Autodesk Inventor part; units mm, degrees
ref_plane "YZ Plane" through (0, 0, 0) normal (1, 0, 0) x (0, 1, 0)
ref_plane "XZ Plane" through (0, 0, 0) normal (0, 1, 0) x (-1, 0, 0)
ref_plane "XY Plane" through (0, 0, 0) normal (0, 0, 1) x (1, 0, 0)
sketch "Sketch1" plane through (0, 0, 0) normal (0, 0, 1) x (1, 0, 0)
  line L0 (-4.7625, -2.7496) -> (-4.7625, 2.7496)
  line L1 (-4.7625, 2.7496) -> (0, 5.4993)
  line L2 (0, 5.4993) -> (4.7625, 2.7496)
  line L3 (4.7625, 2.7496) -> (4.7625, -2.7496)
  line L4 (4.7625, -2.7496) -> (0, -5.4993)
  line L5 (0, -5.4993) -> (-4.7625, -2.7496)
  point P0 (0, 0)
  point P1 (0, 0)
  dimension "Size" = 9.525
extrude "Extrusion1" add sketch "Sketch1" along normal mid plane 66.294
sketch "Sketch3" plane through (0, 0, 33.147) normal (0, 0, 1) x (1, 0, 0)
  line L0 (-4.7625, 2.7496) -> (0, 5.4993) construction
  line L1 (0, 5.4993) -> (4.7625, 2.7496) construction
  line L2 (4.7625, 2.7496) -> (4.7625, -2.7496) construction
  line L3 (4.7625, -2.7496) -> (0, -5.4993) construction
  line L4 (0, -5.4993) -> (-4.7625, -2.7496) construction
  line L5 (-4.7625, -2.7496) -> (-4.7625, 2.7496) construction
  point P0 (0, 0)
hole "Hole1" at (0, 0, 33.147) direction (0, 0, -1) diameter 4.4958 end through all
sketch "Sketch4" plane through (0, 0, 33.147) normal (0, 0, 1) x (1, 0, 0)
  circle A0 centre (0, 0) radius 2.2479 construction
  line L0 (-4.7625, 2.7496) -> (0, 5.4993) construction
  line L1 (0, 5.4993) -> (4.7625, 2.7496) construction
  line L2 (4.7625, 2.7496) -> (4.7625, -2.7496) construction
  line L3 (4.7625, -2.7496) -> (0, -5.4993) construction
  line L4 (0, -5.4993) -> (-4.7625, -2.7496) construction
  line L5 (-4.7625, -2.7496) -> (-4.7625, 2.7496) construction
  circle A1 centre (0, 0) radius 5.1245
  circle A2 centre (0, 0) radius 8.89
  dimension "thunder" = 10.2489
  dimension "d16" = 17.78
extrude "Extrusion3" cut sketch "Sketch4" against normal through all
sketch "Sketch5" plane through (0, 0, 33.147) normal (0, 0, 1) x (1, 0, 0)
  circle A0 centre (0, 0) radius 2.2479
  circle A1 centre (0, 0) radius 4.7625
  line L0 (4.7625, -1.8917) -> (4.7625, 1.8917)
  line L1 (4.0195, 3.1786) -> (0.743, 5.0703)
  line L2 (-0.743, 5.0703) -> (-4.0195, 3.1786)
  line L3 (-4.7625, 1.8917) -> (-4.7625, -1.8917)
  line L4 (-4.0195, -3.1786) -> (-0.743, -5.0703)
  line L5 (0.743, -5.0703) -> (4.0195, -3.1786)
  circle A2 centre (0, 0) radius 2.2479
  arc A3 (4.0195, -3.1786) -> (4.7625, -1.8917) centre (0, 0) ccw
  arc A4 (4.7625, 1.8917) -> (4.0195, 3.1786) centre (0, 0) ccw
  arc A5 (0.743, 5.0703) -> (-0.743, 5.0703) centre (0, 0) ccw
  arc A6 (-4.0195, 3.1786) -> (-4.7625, 1.8917) centre (0, 0) ccw
  arc A7 (-4.7625, -1.8917) -> (-4.0195, -3.1786) centre (0, 0) ccw
  arc A8 (-0.743, -5.0703) -> (0.743, -5.0703) centre (0, 0) ccw
  point P0 (2.3813, -4.1244)
  point P1 (-2.3813, -4.1244)
  point P2 (-4.7625, 0)
  point P3 (-2.3813, 4.1244)
  point P4 (2.3812, 4.1244)
  point P5 (4.7625, 0)
  dimension "d21" = 9.525
extrude "Extrusion4" cut sketch "Sketch5" against normal blind 7.9248 contours L0 A3 L5 A1 | A1 L1 A4 L0 | A1 L2 A5 L1 | L5 A8 L4 A1 | A1 L3 A6 L2 | L4 A7 L3 A1
mirror "Mirror2" about plane through (0, 0, 0) normal (0, 0, 1) of "Extrusion4"
equation "\"bearing\" = 25.4"
properties part number "GP9-008" material "Aluminum 6061"
Work out the finished part from the listing and answer in its coordinate system (mm). A direction names the side the tool comes from. Round coordinates to 2 decimals unless told otherwise and drop trailing zeros. Write each loop counter-clockwise with the first axis right and the second up, starting at its lowest first coordinate (ties: lowest second). Pieces come first, ordered by that corner, then holes. Notation, with made-up numbers: M 32.25,21.5 L 75.25,21.5 A13 cw 75.25,40.5 Z; hole C -32.75,8 d9. An arc over 180 degrees is marked long. Use a Markdown table: item, result.
1) The part is cut by section A-A on x = 0. Give the vertices of the cut face in (y, z).
Taken from the geometry:
| item | result |
|---|---|
| outline | M -5.12,-25.22 L -4.76,-25.22 L -4.76,-33.15 L -2.25,-33.15 L -2.25,33.15 L -4.76,33.15 L -4.76,25.22 L -5.12,25.22 Z; M 2.25,-33.15 L 4.76,-33.15 L 4.76,-25.22 L 5.12,-25.22 L 5.12,25.22 L 4.76,25.22 L 4.76,33.15 L 2.25,33.15 Z |
2) Consider line 1 (X direction, y = -0.25, z = -2.5); line 2 (Z direction, x = 4, y = 3); line 3 (Y direction, x = -1, z = -26). Determine where each line is inside the solid, lowest interval first. Write a range as [from, to].
Taken from the geometry:
| item | result |
|---|---|
| line 1 | x = [-4.76, -2.23], [2.23, 4.76] |
| line 2 | z = [-25.22, 25.22] |
| line 3 | y = [-4.66, -2.01], [2.01, 4.66] |
3) The part is cut by section C-C on z = -5. Give the vertices of the cut face in (x, y), plus the area to 3 significant figures.
Taken from the geometry:
| item | result |
|---|---|
| outline | M -4.76,-1.89 A5.12 ccw -4.02,-3.18 L -0.74,-5.07 A5.12 ccw 0.74,-5.07 L 4.02,-3.18 A5.12 ccw 4.76,-1.89 L 4.76,1.89 A5.12 ccw 4.02,3.18 L 0.74,5.07 A5.12 ccw -0.74,5.07 L -4.02,3.18 A5.12 ccw -4.76,1.89 Z; hole C 0,0 d4.5 |
| area | 61.1 mm2 |
4) Which of the six approach directions +Z, -Z, +X, -X, +Y, -Y give full straight-line access (tool end or side, diameter ignored) to faces 1 (the face through (4.3, -2.5, 25.222)), 2 (the face through (4.3, 2.4, -25.222)), 3 (the face through (4.3, 2.4, 25.222)), 4 (the face through (4.3, -2.5, -25.222))?
Taken from the geometry:
| item | result |
|---|---|
| face 1 | +Z, +X, -Y |
| face 2 | -Z, +X, +Y |
| face 3 | +Z, +X, +Y |
| face 4 | -Z, +X, -Y |
5) Flat-ended cylindrical pins translate along their axes: pin 1 (2 mm diameter, centred on x = -3, z = -7, fed in from +Y); pin 2 (2 mm diameter, centred on x = -2, z = -25, fed in from +Y). Find the tip coordinate at first contact, or state that the pin passes through.
Taken from the geometry:
| item | result |
|---|---|
| pin 1 | stops at y = 4.34 |
| pin 2 | stops at y = 4.92 |
6) Determine the mould class of faces 5 (the face through (-3.78, 2.9, -29.24)), 6 (the face through (-4.3, -2.5, 25.222)), 7 (the face through (4.433, -2.571, 0.353)), 8 (the face through (0.861, -2.076, -0.464)) for opening direction X: pulls with the +X half, pulls with the -X half, needs draft (parallel to the pull), parting line crosses it, or undercut.
Taken from the geometry:
| item | result |
|---|---|
| face 5 | parting line crosses it |
| face 6 | needs draft |
| face 7 | pulls with the +X half |
| face 8 | undercut |
7) The part is cut by section B-B on y = -0.75. Give the vertices of the cut face in (x, z).
Taken from the geometry:
| item | result |
|---|---|
| outline | M -4.76,-25.22 L -4.7,-25.22 L -4.7,-33.15 L -2.12,-33.15 L -2.12,33.15 L -4.7,33.15 L -4.7,25.22 L -4.76,25.22 Z; M 2.12,-33.15 L 4.7,-33.15 L 4.7,-25.22 L 4.76,-25.22 L 4.76,25.22 L 4.7,25.22 L 4.7,33.15 L 2.12,33.15 Z |
8) The part is cut by section D-D on x = 3. Give the vertices of the cut face in (y, z).
Taken from the geometry:
| item | result |
|---|---|
| outline | M -3.77,-25.22 L -3.7,-25.22 L -3.7,-33.15 L 3.7,-33.15 L 3.7,-25.22 L 3.77,-25.22 L 3.77,25.22 L 3.7,25.22 L 3.7,33.15 L -3.7,33.15 L -3.7,25.22 L -3.77,25.22 Z |
